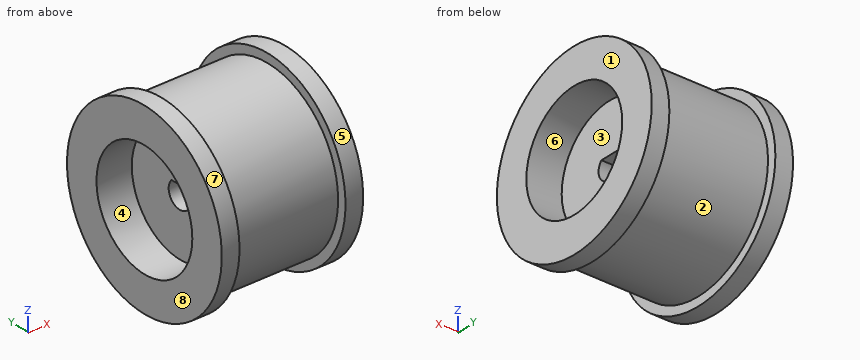
```python
from build123d import *

# Parameters (mm, degrees)
CUT_EXTRUDE1_DEPTH = 10


with BuildPart() as part:
    # Sketch1 → Revolve1 (revolve)
    with BuildSketch(Plane.XY):
        Polygon((6, 9.5), (-6, 9.5), (-6, 10.5), (-8, 10.5), (-8, 6.5), (-4, 6.5), (-4, 0), (4, 0), (4, 6.5), (8, 6.5), (8, 10.5), (6, 10.5), align=None)
    revolve(axis=Axis((-167.001765705, 0, 0), (1, 0, 0)))

    # Sketch2 → Cut-Extrude1 (cut)
    with BuildSketch(Plane(origin=(4, 0, 0), x_dir=(0, 0, -1), z_dir=(1, 0, 0))):
        with BuildLine():
            Line((-1, 1.118033989), (-1, -1.118033989))
            ThreePointArc((-1, -1.118033989), (1.5, 0), (-1, 1.118033989))
        make_face()
    extrude(amount=-CUT_EXTRUDE1_DEPTH, mode=Mode.SUBTRACT)


solid = part.part
```
Can you work these out from the model? Positions are in its coordinate system, mm. Face numbers are marked on the shaded views. A direction names the side the tool comes from. Give positions to 0.01 mm unless a question says otherwise; leave off trailing zeros. Loops run counter-clockwise (first coordinate to the right, second up) from the corner with the lowest first, then second, coordinate; pieces in that order, holes last. Notation, with made-up numbers: M 8.5,-22 L 15.5,-22 A25 ccw 15.5,-1 Z; hole C -10.5,-35.75 d7. An arc over 180 degrees is marked long. One line per item, written item: value.
(1) Will these pins go through, and if not, where does the flat tip stop? pin 1 (5 mm diameter, centred on x = 3, y = 3.5, fed in from -Z); pin 2 (12 mm diameter, centred on y = 3, z = 2, fed in from +X); pin 3 (2 mm diameter, centred on x = 3, z = 4.5, fed in from +Y); pin 4 (4 mm diameter, centred on y = -3, z = 0.5, fed in from +X).
Returned:
pin 1: z = -9.45
pin 2: x = 8
pin 3: y = 8.83
pin 4: x = 4
(2) I need wall thicknesses on line 1 (Z direction, x = -5.4, y = 0); line 2 (Z direction, x = 6.5, y = 0); line 3 (X direction, y = 9.75, z = 0). Which ranges of each line are inside material? Lowest first, please.
Returned:
line 1: -9.5 to -6.5, 6.5 to 9.5
line 2: -10.5 to -6.5, 6.5 to 10.5
line 3: -8 to -6, 6 to 8
(3) Suppose I cut it at A-A on z = 0. List the corners of the cut face in (x, y) for me.
Returned:
outline: M -8,-10.5 L -6,-10.5 L -6,-9.5 L 6,-9.5 L 6,-10.5 L 8,-10.5 L 8,-6.5 L 4,-6.5 L 4,-1.5 L -4,-1.5 L -4,-6.5 L -8,-6.5 Z; M -8,6.5 L -4,6.5 L -4,1.5 L 4,1.5 L 4,6.5 L 8,6.5 L 8,10.5 L 6,10.5 L 6,9.5 L -6,9.5 L -6,10.5 L -8,10.5 Z
(4) We'd pull the mould along Y, two halves only. Please class the marked faces 6, 7 and 8: released by +Y, released by -Y, zero draft, split by the parting line, or undercut.
Returned:
face 6: undercut
face 7: split by the parting line
face 8: zero draft
(5) Suppose I cut it at B-B on y = 0. List the corners of the cut face in (x, z) for me, plus the area to 3 significant figures.
Returned:
outline: M -8,-10.5 L -6,-10.5 L -6,-9.5 L 6,-9.5 L 6,-10.5 L 8,-10.5 L 8,-6.5 L 4,-6.5 L 4,-1.5 L -4,-1.5 L -4,-6.5 L -8,-6.5 Z; M -8,6.5 L -4,6.5 L -4,1 L 4,1 L 4,6.5 L 8,6.5 L 8,10.5 L 6,10.5 L 6,9.5 L -6,9.5 L -6,10.5 L -8,10.5 Z
area: 188 mm^2
(6) Suppose I cut it at C-C on x = 2. List the corners of the cut face in (y, z) for me, plus the area to 3 significant figures.
Returned:
outline: C 0,0 d19; hole M -1.12,1 A1.5 ccw long 1.12,1 Z
area: 277 mm^2
(7) Which directions (+Z, -Z, +X, -X, +Y, -Y) give clear straight access to the entire face, cutting with the end or side of a thin tool? Please do the marked faces 1, 2, 3, 4 and 5.
Returned:
face 1: +Z, -Z, +X, +Y, -Y
face 2: none
face 3: +X
face 4: -X
face 5: +X, -X
(8) Suppose I cut it at D-D on y = -2.5. List the corners of the cut face in (x, z) for me.
Returned:
outline: M -8,-10.2 L -6,-10.2 L -6,-9.17 L 6,-9.17 L 6,-10.2 L 8,-10.2 L 8,-6 L 4,-6 L 4,6 L 8,6 L 8,10.2 L 6,10.2 L 6,9.17 L -6,9.17 L -6,10.2 L -8,10.2 L -8,6 L -4,6 L -4,-6 L -8,-6 Z
